Verification items for the finished model (mm, model axes). A direction names the side the tool comes from. Coordinates: 2 decimals unless noted, no trailing zeros. Loops run counter-clockwise (first coordinate to the right, second up) from the corner with the lowest first, then second, coordinate; pieces in that order, holes last.
Q1. Access from +Z, -Z, +X, -X, +Y, -Y to the whole of each face (thin tool, end or side, straight path). Record for faces 1 (the face through (-3, 0.8, 2)), 2 (the face through (-1.739, 0.394, 2.465)), 3 (the face through (1.5, 4.2, 5)).
Q2. Sectioned sample at B-B (y = 7.75). Enter the section's corners in (x, z).
Q3. Mould release check, pull along X, two halves, no side actions. Record for faces 4 (the face through (-1, 0, 2)), 5 (the face through (-2, -3, 2)), 6 (the face through (-4, 9, 2)): +X half, -X half, draft (parallel to the pull), parting line (faces both ways), or undercut.
Q4. Material ranges on probe 1 along Y at (x, z) = (-1, 0.5); probe 2 along Y at (x, z) = (1.5, 4.35); probe 3 along X at (y, z) = (9.5, 3.4), recorded low to high.
Q5. Sectioned sample at C-C (z = 3.6). Enter the section's corners in (x, y), then the cut area to 3 significant figures.
Q6. Sectioned sample at A-A (x = -0.25). Enter the section's corners in (y, z).
Q7. Go/stop test with flat-tipped pins: P1, Ø4, axis at x = 0.5, y = 0.5, coming from the -Z side; P2, Ø1.5, axis at x = 3.5, z = 4, coming from the +Y side. Record where each tip stops, or that it passes through.
Q8. Sectioned sample at D-D (x = 1.75). Enter the section's corners in (y, z).
```python
from build123d import *

# Parameters (mm, degrees)
F1_DEPTH = 5
F2_SIZE  = 1
F3_R     = 0.5


with BuildPart() as f1:
    # F0 (on Top) → F1 (new body)
    with BuildSketch(Plane.XY):
        with BuildLine():
            ThreePointArc((0, 8.2), (1.449569, 7.599569), (2.05, 6.15))
            Line((2.05, 6.15), (2.05, 5.1))
            Line((2.05, 5.1), (2.05, 4.1))
            Line((2.05, 4.1), (2.05, 3.1))
            Line((2.05, 3.1), (2.05, 2.05))
            ThreePointArc((2.05, 2.05), (1.449569, 0.600431), (0, 0))
            Line((0, 0), (-1.344113, 0))
            Line((-1.344113, 0), (-4, 0))
            Line((-4, 0), (-4, -3))
            Line((-4, -3), (0, -3))
            ThreePointArc((0, -3), (3.570889, -1.520889), (5.05, 2.05))
            Line((5.05, 2.05), (5.05, 6.15))
            ThreePointArc((5.05, 6.15), (3.570889, 9.720889), (0, 11.2))
            Line((0, 11.2), (-4, 11.2))
            Line((-4, 11.2), (-4, 8.2))
            Line((-4, 8.2), (-1.344113, 8.2))
            Line((-1.344113, 8.2), (0, 8.2))
        make_face()
        Polygon((-2.144113, 7.4), (-1.344113, 8.2), (-4, 8.2), (-3.2, 7.4), align=None)
        Polygon((-3.2, 0.8), (-4, 0), (-1.344113, 0), (-2.144113, 0.8), align=None)
        Polygon((2.05, 4.1), (2.05, 5.1), (1.05, 4.1), align=None)
        Polygon((2.05, 3.1), (2.05, 4.1), (1.05, 4.1), align=None)
    extrude(amount=F1_DEPTH)

    # F2
    f2_edges = [f1.edges().sort_by_distance(p)[0] for p in [
        (-4, 11.2, 2.5),
        (-4, -3, 2.5),
    ]]
    chamfer(f2_edges, length=F2_SIZE)

    # F3
    f3_edges = [f1.edges().sort_by_distance(p)[0] for p in [
        (1.05, 4.1, 2.5),
    ]]
    fillet(f3_edges, radius=F3_R)


solid = f1.part
```
Geometry check:
1. face 1: +Z, -Z, -X
1. face 2: +Z, -Z
1. face 3: +Z, +X, -X, +Y, -Y
2. outline: (-3.55, 0) - (-1.79, 0) - (-1.79, 5) - (-3.55, 5) - close; (1.28, 0) - (4.79, 0) - (4.79, 5) - (1.28, 5) - close
3. face 4: undercut
3. face 5: draft
3. face 6: -X half
4. probe 1: y = -3 to 0, 8.2 to 11.2
4. probe 2: y = -2.77 to 0.65, 3.65 to 4.55, 7.55 to 10.97
4. probe 3: x = -4 to 3.78
5. outline: (-4, -2) - (-3, -3) - (0, -3) arc R5.05 ccw to (5.05, 2.05) - (5.05, 6.15) arc R5.05 ccw to (0, 11.2) - (-3, 11.2) - (-4, 10.2) - (-4, 8.2) - (-3.2, 7.4) - (-2.14, 7.4) - (-1.34, 8.2) - (0, 8.2) arc R2.05 cw to (2.05, 6.15) - (2.05, 5.1) - (1.4, 4.45) arc R0.5 ccw to (1.4, 3.75) - (2.05, 3.1) - (2.05, 2.05) arc R2.05 cw to (0, 0) - (-1.34, 0) - (-2.14, 0.8) - (-3.2, 0.8) - (-4, 0) - close
5. area: 72.7 mm2
6. outline: (-3, 0) - (0, 0) - (0, 5) - (-3, 5) - close; (8.2, 0) - (11.2, 0) - (11.2, 5) - (8.2, 5) - close
7. P1: stops at z = 0
7. P2: stops at y = 10.39
8. outline: (-2.69, 0) - (0.98, 0) - (0.98, 5) - (-2.69, 5) - close; (3.4, 0) - (4.8, 0) - (4.8, 5) - (3.4, 5) - close; (7.22, 0) - (10.89, 0) - (10.89, 5) - (7.22, 5) - close
